The model under review builds one solid part; all positions refer to its coordinate system, in mm. Round coordinates to 2 decimals unless told otherwise and drop trailing zeros. Write each loop counter-clockwise with the first axis right and the second up, starting at its lowest first coordinate (ties: lowest second). Pieces come first, ordered by that corner, then holes. Notation, with made-up numbers: (82, -15) - (132, -15) arc R16 ccw to (132, 6) - close; hole circle Ø6 at (87, -38). An arc over 180 degrees is marked (long way). One line per question, with ' | ' between items. Start each with the question number.
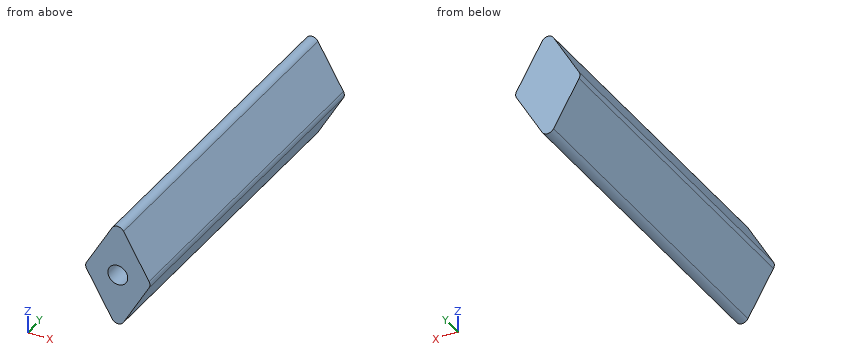
```python
from build123d import *

# Parameters (mm, degrees)
BOSS_EXTRUDE1_DEPTH = 52
CUT_EXTRUDE1_DEPTH  = 45
SKETCH3_R           = 1.5
CUT_EXTRUDE2_DEPTH  = 8
BOSS_EXTRUDE2_DEPTH = 1
CUT_EXTRUDE5_DEPTH  = 10
FILLET1_R           = 1


with BuildPart() as part:
    # Sketch1 → Boss-Extrude1 (new body)
    with BuildSketch(Plane(origin=(0, 0, 0), x_dir=(1, 0, 0), z_dir=(0, 1, 0))):
        Polygon((-5, 0), (0, 8.660254), (5, 0), (0, -8.660254), align=None)
    extrude(amount=-BOSS_EXTRUDE1_DEPTH)

    # Sketch2 → Cut-Extrude1 (cut)
    with BuildSketch(Plane(origin=(0, 0, 0), x_dir=(1, 0, 0), z_dir=(0, 1, 0))):
        Polygon((0, 6.660254), (-3.845299, 0), (0, -6.660254), (3.845299, 0), align=None)
    extrude(amount=-CUT_EXTRUDE1_DEPTH, mode=Mode.SUBTRACT)

    # Sketch3 → Cut-Extrude2 (cut, through all)
    with BuildSketch(Plane(origin=(0, -45, 0), x_dir=(1, 0, 0), z_dir=(0, 1, 0))):
        Circle(SKETCH3_R)
    extrude(amount=-CUT_EXTRUDE2_DEPTH, mode=Mode.SUBTRACT)

    # Sketch5 → Boss-Extrude2 (add)
    with BuildSketch(Plane(origin=(0, 0, 0), x_dir=(1, 0, 0), z_dir=(0, 1, 0))):
        Polygon((-3.845299, 0), (0, 6.660254), (3.845299, 0), (0, -6.660254), align=None)
    extrude(amount=-BOSS_EXTRUDE2_DEPTH)

    # Sketch12 → Cut-Extrude5 (cut)
    with BuildSketch(Plane.XZ.offset(52)):
        with BuildLine():
            Line((-0.866025, 7.160254), (0, 8.660254))
            Line((0, 8.660254), (0.866025, 7.160254))
            ThreePointArc((0.866025, 7.160254), (0, 7.660254), (-0.866025, 7.160254))
        make_face()
        with BuildLine():
            Line((-4.711325, 0.5), (-5, 0))
            Line((-5, 0), (-4.711325, -0.5))
            ThreePointArc((-4.711325, -0.5), (-4.845299, 0), (-4.711325, 0.5))
        make_face()
        with BuildLine():
            Line((-0.866025, -7.160254), (0, -8.660254))
            Line((0, -8.660254), (0.866025, -7.160254))
            ThreePointArc((0.866025, -7.160254), (0, -7.660254), (-0.866025, -7.160254))
        make_face()
        with BuildLine():
            Line((4.711325, 0.5), (5, 0))
            Line((5, 0), (4.711325, -0.5))
            ThreePointArc((4.711325, -0.5), (4.845299, 0), (4.711325, 0.5))
        make_face()
    extrude(amount=-CUT_EXTRUDE5_DEPTH, mode=Mode.SUBTRACT)

    # Fillet1
    fillet1_edges = [part.edges().sort_by_distance(p)[0] for p in [
        (-5, -21, 0),
        (0, -21, 8.660254),
        (5, -21, 0),
        (0, -21, -8.660254),
    ]]
    fillet(fillet1_edges, radius=FILLET1_R)


solid = part.part
```
1. Add section A-A, the plane y = -24.5. Write out the cut boundary in (x, z), then the cut area to 3 significant figures.
2. Add section C-C, the plane x = -2.75. Write out the cut boundary in (y, z).
3. Add section B-B, the plane z = -5.5. Write out the cut boundary in (x, y).
4. Wall thickness on line 1 along X through (y, z) = (-48.5, 0); line 2 along Y through (x, z) = (0, -2.5); line 3 along Z through (x, y) = (-0.75, -48): over which ranges is each line inside the solid? List them lowest first. Write a range as [from, to].
5. Add section D-D, the plane z = 1. Write out the cut boundary in (x, y).
6. Clearance check with a flat-ended pin moving along its axis: P1, Ø2.5, axis at x = 0, z = 0, coming from the -Y side. State where the tip first meets the part, or that it passes through.
Geometry check:
1) outline: (-4.71, -0.5) - (-0.87, -7.16) arc R1 ccw to (0.87, -7.16) - (4.71, -0.5) arc R1 ccw to (4.71, 0.5) - (0.87, 7.16) arc R1 ccw to (-0.87, 7.16) - (-4.71, 0.5) arc R1 ccw to start; hole (-3.85, 0) - (0, -6.66) - (3.85, 0) - (0, 6.66) - close | area: 33.9 mm2
2) outline: (-52, -3.9) - (0, -3.9) - (0, 3.9) - (-52, 3.9) - close; hole (-45, -1.9) - (-1, -1.9) - (-1, 1.9) - (-45, 1.9) - close
3) outline: (-1.82, -52) - (1.82, -52) - (1.82, 0) - (-1.82, 0) - close; hole (-0.67, -45) - (0.67, -45) - (0.67, -1) - (-0.67, -1) - close
4) line 1: x = [-4.85, -1.5], [1.5, 4.85] | line 2: y = [-52, -45], [-1, 0] | line 3: z = [-7.32, -1.3], [1.3, 7.32]
5) outline: (-4.42, -52) - (-1.12, -52) - (-1.12, -45) - (-3.27, -45) - (-3.27, -1) - (3.27, -1) - (3.27, -45) - (1.12, -45) - (1.12, -52) - (4.42, -52) - (4.42, 0) - (-4.42, 0) - close
6) P1: stops at y = -1
